Design review of the part shown in the three views and the two pictorial views. Dimensions are in mm from the part's minimum x, y and z. Round coordinates to 2 decimals unless told otherwise and drop trailing zeros. Write each loop counter-clockwise with the first axis right and the second up, starting at its lowest first coordinate (ties: lowest second). Pieces come first, ordered by that corner, then holes. Notation, with made-up numbers: (-12.75, 33.5) - (20.25, 33.5) arc R23 cw to (20.25, 44.5) - close; hole circle Ø10 at (-20.5, 10). An arc over 180 degrees is marked (long way). One line per item, written item: value. Start each with the question number.
Q1. Add section A-A on z = 13. Give the number of separate pieces and of enclosed holes in the cut face, and give its area (3 significant figures).
Q2. Add section B-B on x = 16. Write out the cut boundary in (y, z), and give its area (3 significant figures).
Q3. Add section C-C on y = 6.25. Write out the cut boundary in (x, z).
Q4. For probe 1 along Z at (x, y) = (13.5, 9); probe 2 along Y at (x, z) = (12.5, 11.25), list the stretches that pass through material, from the lowest coordinate up.
Q5. Clearance check with flat-ended pins moving along their axes: pin 1 Ø6 at (y, z) = (4.5, 12) entering from -X; pin 2 Ø1.5 at (x, y) = (26.5, 8.5) entering from +Z. State where each tip first meets the part, or that it passes through.
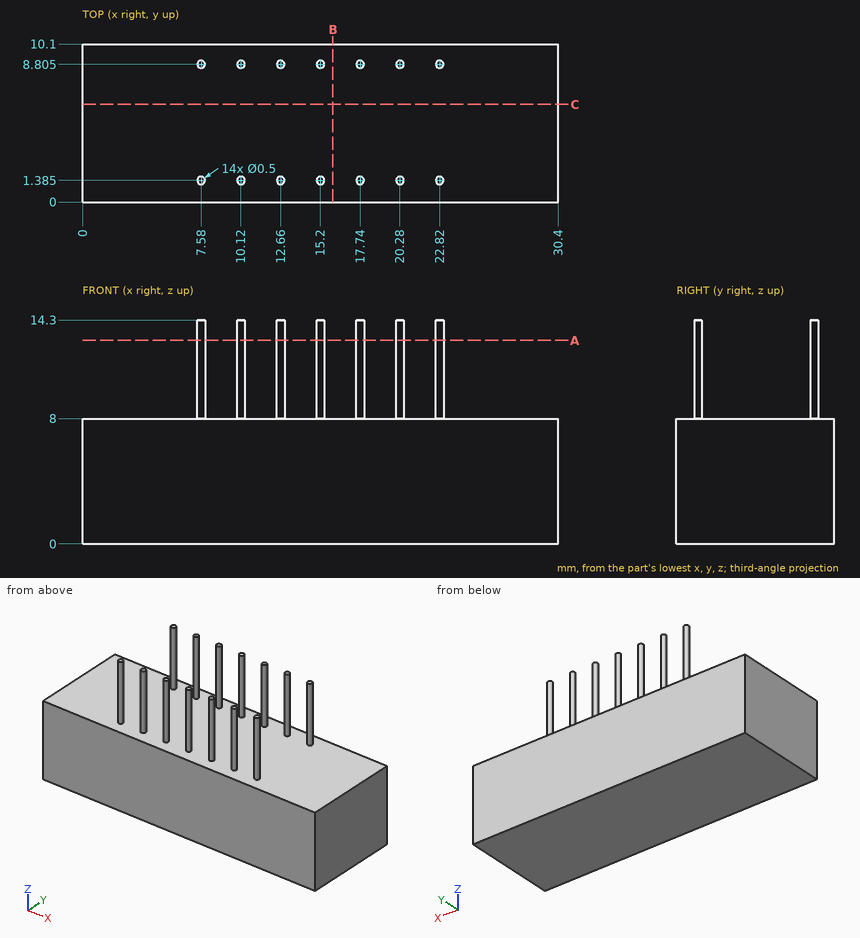
Result set:
1. separate pieces: 14
1. enclosed holes: 0
1. area: 2.75 mm^2
2. outline: (0, 0) - (10.1, 0) - (10.1, 8) - (0, 8) - close
2. area: 80.8 mm^2
3. outline: (0, 0) - (30.4, 0) - (30.4, 8) - (0, 8) - close
4. probe 1: z = 0 to 8
4. probe 2: y = 1.19 to 1.58, 8.61 to 9
5. pin 1: stops at x = 7.36
5. pin 2: stops at z = 8
